Verification items for the finished model (mm, model axes). A direction names the side the tool comes from. Coordinates: 2 decimals unless noted, no trailing zeros. Write each loop counter-clockwise with the first axis right and the second up, starting at its lowest first coordinate (ties: lowest second). Pieces come first, ordered by that corner, then holes. Notation, with made-up numbers: (9, 20.5) -> (54, 20.5) arc R17 ccw to (54, 44.5) -> close; hole circle Ø9 at (15.5, 86.5). An arc over 180 degrees is marked (long way). Write item = value, one per line. Start each with the question number.
(1) Gauge pin test, flat ends, axial feed: pin 1 Ø7 at (y, z) = (0, -50) entering from -X; pin 2 Ø2.5 at (x, z) = (33, 105) entering from -Y; pin 3 Ø1.5 at (y, z) = (-107.5, -86) entering from +X; pin 4 Ø6.5 at (y, z) = (71.5, 123.84) entering from +X. Record the tip position at first contact, or that the pin passes through.
(2) Material ranges on probe 1 along Z at (x, y) = (1296.5, -111.5); probe 2 along Y at (x, z) = (1593, 0); probe 3 along X at (y, z) = (-93, -91), recorded low to high. Write a range as [from, to].
(3) Mould release check, pull along Z, two halves, no side actions. Record for faces 1 (the face through (-20, 0, 0)), 2 (the face through (801, -110, -100)), 3 (the face through (801, -105, 10)): released by +Z, released by -Z, zero draft, split by the parting line, or undercut.
(4) Set-up check for faces 4 (the face through (20.14, -19.524, 4.336)), 5 (the face through (1594.93, 2.64, 59.94)), 6 (the face through (40, 13, 5)): record each of +Z, -Z, +X, -X, +Y, -Y from which the full face is reachable in a straight line by a thin tool's end or side.
(5) Section check A-A (x = 1496.5). Record the cut outline in (y, z).
```python
from build123d import *

# Parameters (mm, degrees)
SKETCH_1_R             = 175
SKETCH_1_R_2           = 5.5
EXTRUDE_1_DEPTH        = 10
SKETCH_2_R             = 20
EXTRUDE_2_DEPTH        = 30
EXTRUDE_START          = 20
SKETCH_2_2_R           = 20
EXTRUDE_3_DEPTH        = 20
SKETCH_3_W             = 10
SKETCH_3_H             = 169.24993674
EXTRUDE_1_2_DEPTH      = 10
SKETCH_4_W             = 1540
SKETCH_4_H             = 10
EXTRUDE_2_2_DEPTH      = 10
PATTERN_LINEAR_1_COUNT = 2
PATTERN_LINEAR_1_PITCH = 1540
PATTERN_LINEAR_2_COUNT = 2
PATTERN_LINEAR_2_PITCH = 1560
SKETCH_5_R             = 60
EXTRUDE_4_DEPTH        = 10
CUT_EXTRUDE_2_REACH    = 1640.795
SKETCH_6_R             = 4.5
SKETCH_7_R             = 12.5
CUT_EXTRUDE_3_DEPTH    = 10
SKETCH_8_W             = 200
SKETCH_8_H             = 10
EXTRUDE_3_2_DEPTH      = 10
PATTERN_LINEAR_4_COUNT = 2
PATTERN_LINEAR_4_PITCH = 1540
SKETCH_9_W             = 10
SKETCH_9_H             = 170
EXTRUDE_4_2_DEPTH      = 10
PATTERN_LINEAR_6_COUNT = 2
PATTERN_LINEAR_6_PITCH = 100
PATTERN_LINEAR_7_COUNT = 2
PATTERN_LINEAR_7_PITCH = 1540
SKETCH_10_W            = 10
SKETCH_10_H            = 170
EXTRUDE_5_DEPTH        = 10
PATTERN_LINEAR_8_COUNT = 2
PATTERN_LINEAR_8_PITCH = 100
PATTERN_LINEAR_9_COUNT = 2
PATTERN_LINEAR_9_PITCH = 1540


with BuildPart() as part:
    # 草图1 → Extrude 1 (new body)
    with BuildSketch(Plane(origin=(0, 0, 0), x_dir=(0, 0, -1), z_dir=(1, 0, 0))):
        Circle(SKETCH_1_R)
        with Locations((-143, 0)):
            Circle(SKETCH_1_R_2, mode=Mode.SUBTRACT)
        with Locations((-123.841632741, 71.5)):
            Circle(SKETCH_1_R_2, mode=Mode.SUBTRACT)
        with Locations((-71.5, 123.841632741)):
            Circle(SKETCH_1_R_2, mode=Mode.SUBTRACT)
        with Locations((0, 143)):
            Circle(SKETCH_1_R_2, mode=Mode.SUBTRACT)
        with Locations((71.5, 123.841632741)):
            Circle(SKETCH_1_R_2, mode=Mode.SUBTRACT)
        with Locations((123.841632741, 71.5)):
            Circle(SKETCH_1_R_2, mode=Mode.SUBTRACT)
        with Locations((143, 0)):
            Circle(SKETCH_1_R_2, mode=Mode.SUBTRACT)
        with Locations((123.841632741, -71.5)):
            Circle(SKETCH_1_R_2, mode=Mode.SUBTRACT)
        with Locations((71.5, -123.841632741)):
            Circle(SKETCH_1_R_2, mode=Mode.SUBTRACT)
        with Locations((0, -143)):
            Circle(SKETCH_1_R_2, mode=Mode.SUBTRACT)
        with Locations((-71.5, -123.841632741)):
            Circle(SKETCH_1_R_2, mode=Mode.SUBTRACT)
        with Locations((-123.841632741, -71.5)):
            Circle(SKETCH_1_R_2, mode=Mode.SUBTRACT)
    extrude(amount=EXTRUDE_1_DEPTH)

    # 草图2 → Extrude 2 (add)
    with BuildSketch(Plane(origin=(10, 0, 0), x_dir=(0, 0, -1), z_dir=(1, 0, 0))):
        Circle(SKETCH_2_R)
    extrude(amount=-EXTRUDE_2_DEPTH)

    # 草图2<2> → Extrude 3 (add)
    with BuildSketch(Plane(origin=(10, 0, 0), x_dir=(0, 0, -1), z_dir=(1, 0, 0)).offset(EXTRUDE_START)):
        Circle(SKETCH_2_2_R)
    extrude_3 = extrude(amount=-EXTRUDE_3_DEPTH)

    # 草图3 → Extrude 1 2 (add)
    with BuildSketch(Plane(origin=(30, 0, 0), x_dir=(0, 0, -1), z_dir=(1, 0, 0))):
        with Locations((-5, -19.147397114)):
            Rectangle(SKETCH_3_W, SKETCH_3_H)
    extrude_1_2 = extrude(amount=EXTRUDE_1_2_DEPTH)

    # 草图4 → Extrude 2 2 (add)
    with BuildSketch(Plane.XY):
        with Locations((805, -108.772365484)):
            Rectangle(SKETCH_4_W, SKETCH_4_H)
    extrude_2_2 = extrude(amount=EXTRUDE_2_2_DEPTH)

    # 阵列(线性)1: Extrude 1 2 ×2
    with Locations(*[(i * PATTERN_LINEAR_1_PITCH, 0, 0) for i in range(1, PATTERN_LINEAR_1_COUNT)]):
        add(extrude_1_2)

    # 阵列(线性)2: Extrude 3 ×2
    with Locations(*[(i * PATTERN_LINEAR_2_PITCH, 0, 0) for i in range(1, PATTERN_LINEAR_2_COUNT)]):
        add(extrude_3)

    # 草图5 → Extrude 4 (add)
    with BuildSketch(Plane(origin=(1590, 0, 0), x_dir=(0, 0, -1), z_dir=(1, 0, 0))):
        Circle(SKETCH_5_R)
    extrude(amount=EXTRUDE_4_DEPTH)

    # 草图6 → 切除-拉伸2 (cut, up to next)
    with BuildSketch(Plane(origin=(1600, 0, 0), x_dir=(0, 0, -1), z_dir=(1, 0, 0)), mode=Mode.PRIVATE) as cut_extrude_2_sk1:
        with Locations((0, 50)):
            Circle(SKETCH_6_R)
    cut_extrude_2_tool1 = extrude(cut_extrude_2_sk1.sketch, amount=-CUT_EXTRUDE_2_REACH, mode=Mode.PRIVATE) & part.part
    # 草图6 → 切除-拉伸2 (cut, up to next)
    with BuildSketch(Plane(origin=(1600, 0, 0), x_dir=(0, 0, -1), z_dir=(1, 0, 0)), mode=Mode.PRIVATE) as cut_extrude_2_sk2:
        with Locations((50, 0)):
            Circle(SKETCH_6_R)
    cut_extrude_2_tool2 = extrude(cut_extrude_2_sk2.sketch, amount=-CUT_EXTRUDE_2_REACH, mode=Mode.PRIVATE) & part.part
    # 草图6 → 切除-拉伸2 (cut, up to next)
    with BuildSketch(Plane(origin=(1600, 0, 0), x_dir=(0, 0, -1), z_dir=(1, 0, 0)), mode=Mode.PRIVATE) as cut_extrude_2_sk3:
        with Locations((0, -50)):
            Circle(SKETCH_6_R)
    cut_extrude_2_tool3 = extrude(cut_extrude_2_sk3.sketch, amount=-CUT_EXTRUDE_2_REACH, mode=Mode.PRIVATE) & part.part
    # 草图6 → 切除-拉伸2 (cut, up to next)
    with BuildSketch(Plane(origin=(1600, 0, 0), x_dir=(0, 0, -1), z_dir=(1, 0, 0)), mode=Mode.PRIVATE) as cut_extrude_2_sk4:
        with Locations((-50, 0)):
            Circle(SKETCH_6_R)
    cut_extrude_2_tool4 = extrude(cut_extrude_2_sk4.sketch, amount=-CUT_EXTRUDE_2_REACH, mode=Mode.PRIVATE) & part.part
    add(cut_extrude_2_tool1.solids().sort_by_distance((1600, 50, 0))[0], mode=Mode.SUBTRACT)
    add(cut_extrude_2_tool2.solids().sort_by_distance((1600, 0, -50))[0], mode=Mode.SUBTRACT)
    add(cut_extrude_2_tool3.solids().sort_by_distance((1600, -50, 0))[0], mode=Mode.SUBTRACT)
    add(cut_extrude_2_tool4.solids().sort_by_distance((1600, 0, 50))[0], mode=Mode.SUBTRACT)

    # 草图7 → 切除-拉伸3 (cut)
    with BuildSketch(Plane(origin=(1600, 0, 0), x_dir=(0, 0, -1), z_dir=(1, 0, 0))):
        Circle(SKETCH_7_R)
    extrude(amount=-CUT_EXTRUDE_3_DEPTH, mode=Mode.SUBTRACT)

    # 草图8 → Extrude 3 2 (add)
    with BuildSketch(Plane(origin=(30, 0, 0), x_dir=(0, 0, -1), z_dir=(1, 0, 0))):
        with Locations((0, 60.477571256)):
            Rectangle(SKETCH_8_W, SKETCH_8_H)
    extrude_3_2 = extrude(amount=EXTRUDE_3_2_DEPTH)

    # 阵列(线性)4: Extrude 3 2 ×2
    with Locations(*[(i * PATTERN_LINEAR_4_PITCH, 0, 0) for i in range(1, PATTERN_LINEAR_4_COUNT)]):
        add(extrude_3_2)

    # 草图9 → Extrude 4 2 (add)
    with BuildSketch(Plane(origin=(30, 0, 0), x_dir=(0, 0, -1), z_dir=(1, 0, 0))):
        with Locations((95, -19.522428744)):
            Rectangle(SKETCH_9_W, SKETCH_9_H)
    extrude_4_2 = extrude(amount=EXTRUDE_4_2_DEPTH)

    # 阵列(线性)6: Extrude 2 2 ×2
    with Locations(*[(0, 0, -i * PATTERN_LINEAR_6_PITCH) for i in range(1, PATTERN_LINEAR_6_COUNT)]):
        add(extrude_2_2)

    # 阵列(线性)7: Extrude 4 2 ×2
    with Locations(*[(i * PATTERN_LINEAR_7_PITCH, 0, 0) for i in range(1, PATTERN_LINEAR_7_COUNT)]):
        add(extrude_4_2)

    # 草图10 → 拉伸-薄壁5 (add)
    with BuildSketch(Plane(origin=(30, 0, 0), x_dir=(0, 0, -1), z_dir=(1, 0, 0))):
        with Locations((-105, -19.522428744)):
            Rectangle(SKETCH_10_W, SKETCH_10_H)
    extrude_5 = extrude(amount=EXTRUDE_5_DEPTH)

    # 阵列(线性)8: Extrude 2 2 ×2
    with Locations(*[(0, 0, i * PATTERN_LINEAR_8_PITCH) for i in range(1, PATTERN_LINEAR_8_COUNT)]):
        add(extrude_2_2)

    # 阵列(线性)9: 拉伸-薄壁5 ×2
    with Locations(*[(i * PATTERN_LINEAR_9_PITCH, 0, 0) for i in range(1, PATTERN_LINEAR_9_COUNT)]):
        add(extrude_5)


solid = part.part
```
Response:
q1.pin_1 = 0
q1.pin_2 = -104.52
q1.pin_3 = 10
q1.pin_4 = through
q2.probe_1 = [-100, -90], [0, 10], [100, 110]
q2.probe_2 = [-60, -54.5], [-45.5, -12.5], [12.5, 45.5], [54.5, 60]
q2.probe_3 = [0, 10], [30, 40], [1570, 1580]
q3.face_1 = zero draft
q3.face_2 = released by -Z
q3.face_3 = undercut
q4.face_4 = none
q4.face_5 = +X
q4.face_6 = +Z, -Z, +Y
q5.outline = (-113.77, -100) -> (-103.77, -100) -> (-103.77, -90) -> (-113.77, -90) -> close; (-113.77, 0) -> (-103.77, 0) -> (-103.77, 10) -> (-113.77, 10) -> close; (-113.77, 100) -> (-103.77, 100) -> (-103.77, 110) -> (-113.77, 110) -> close
